Check sheet for the modelled part. Datum: model origin and axes. Units: mm. Face numbers are marked on the shaded views. A direction names the side the tool comes from. Round coordinates to 2 decimals unless told otherwise and drop trailing zeros. Write each loop counter-clockwise with the first axis right and the second up, starting at its lowest first coordinate (ties: lowest second). Pieces come first, ordered by that corner, then holes. Notation, with made-up numbers: (-36.75, 82) -> (2.25, 82) arc R24 cw to (2.25, 112) -> close; hole circle Ø3 at (51, -33.75). An arc over 180 degrees is marked (long way). Answer as a JSON object with one key per item and string values. Group by question number.
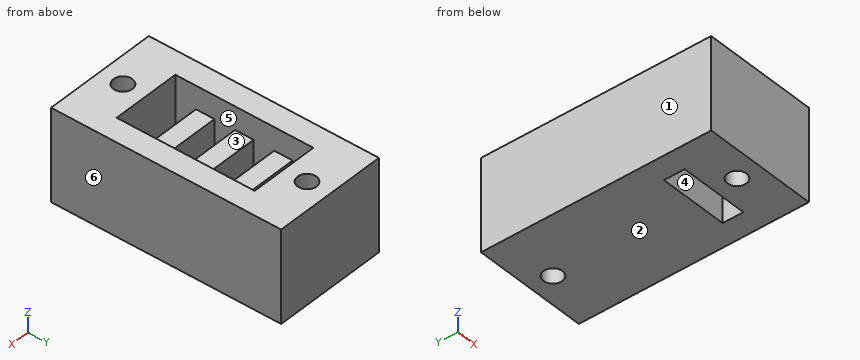
```python
from build123d import *

# Parameters (mm, degrees)
SKETCH1_W           = 12.7
SKETCH1_H           = 10.16
BOSS_EXTRUDE1_DEPTH = 25.4
SKETCH2_W           = 7.62
SKETCH2_H           = 15.24
CUT_EXTRUDE1_DEPTH  = 7.62
SKETCH3_W           = 5.08
SKETCH3_H           = 2.032
BOSS_EXTRUDE2_DEPTH = 7.62
SKETCH4_W           = 7.62
SKETCH4_H           = 2.286
CUT_EXTRUDE2_DEPTH  = 3.54
SKETCH5_R           = 1.0414
CUT_EXTRUDE4_DEPTH  = 11.16


with BuildPart() as part:
    # Sketch1 → Boss-Extrude1 (new body)
    with BuildSketch(Plane(origin=(0, 0, 0), x_dir=(1, 0, 0), z_dir=(0, 1, 0))):
        Rectangle(SKETCH1_W, SKETCH1_H)
    extrude(amount=BOSS_EXTRUDE1_DEPTH)

    # Sketch2 → Cut-Extrude1 (cut)
    with BuildSketch(Plane.XY.offset(5.08)):
        with Locations((0, 12.7)):
            Rectangle(SKETCH2_W, SKETCH2_H)
    extrude(amount=-CUT_EXTRUDE1_DEPTH, mode=Mode.SUBTRACT)

    # Sketch3 → Boss-Extrude2 (add)
    with BuildSketch(Plane.ZY.offset(-3.81)):
        with Locations((0, 12.7)):
            Rectangle(SKETCH3_W, SKETCH3_H)
        with Locations((0, 8.382)):
            Rectangle(SKETCH3_W, SKETCH3_H)
        with Locations((0, 17.018)):
            Rectangle(SKETCH3_W, SKETCH3_H)
    extrude(amount=BOSS_EXTRUDE2_DEPTH)

    # Sketch4 → Cut-Extrude2 (cut, through all)
    with BuildSketch(Plane.XY.offset(-2.54)):
        with Locations((0, 6.223)):
            Rectangle(SKETCH4_W, SKETCH4_H)
    extrude(amount=-CUT_EXTRUDE2_DEPTH, mode=Mode.SUBTRACT)

    # Sketch5 → Cut-Extrude4 (cut, through all)
    with BuildSketch(Plane.XY.offset(5.08)):
        with Locations((0, 2.54)):
            Circle(SKETCH5_R)
        with Locations((0, 22.86)):
            Circle(SKETCH5_R)
    extrude(amount=-CUT_EXTRUDE4_DEPTH, mode=Mode.SUBTRACT)


solid = part.part
```
(1) Section check A-A on x = 0. Record the cut outline in (y, z).
(2) Section check C-C on x = 3.5. Record the cut outline in (y, z), then the cut area to 3 significant figures.
(3) Access from +Z, -Z, +X, -X, +Y, -Y to the whole of each face (thin tool, end or side, straight path). Record for the marked faces 4, 5 and 6.
(4) Section check D-D on y = 2.54. Record the cut outline in (x, z).
(5) Release check for a two-part mould opening along X. For the marked faces 1, 2 and 3 record: pulls with the +X half, pulls with the -X half, needs draft (parallel to the pull), parting line crosses it, or undercut.
(6) Section check B-B on z = -1.25. Record the cut outline in (x, y), then the cut area to 3 significant figures.
(7) Scan lines: line 1 along Y through (x, z) = (0, 3.25); line 2 along Y through (x, z) = (-1.25, 3.5); line 3 along X through (y, z) = (15.5, -1). Record each from-to range of solid material in increasing order.
(8) Go/stop test with a flat-tipped pin: pin 1 Ø1.6 at (x, y) = (-1, 17.5) entering from +Z. Record where the tip stops, or that it passes through.
Data:
{
 "1": {"outline": "(0, -5.08) -> (1.5, -5.08) -> (1.5, 5.08) -> (0, 5.08) -> close; (3.58, -5.08) -> (5.08, -5.08) -> (5.08, 5.08) -> (3.58, 5.08) -> close; (7.37, -5.08) -> (21.82, -5.08) -> (21.82, 5.08) -> (20.32, 5.08) -> (20.32, -2.54) -> (18.03, -2.54) -> (18.03, 2.54) -> (16, 2.54) -> (16, -2.54) -> (13.72, -2.54) -> (13.72, 2.54) -> (11.68, 2.54) -> (11.68, -2.54) -> (9.4, -2.54) -> (9.4, 2.54) -> (7.37, 2.54) -> close; (23.9, -5.08) -> (25.4, -5.08) -> (25.4, 5.08) -> (23.9, 5.08) -> close"},
 "2": {"outline": "(0, -5.08) -> (5.08, -5.08) -> (5.08, 5.08) -> (0, 5.08) -> close; (7.37, -5.08) -> (25.4, -5.08) -> (25.4, 5.08) -> (20.32, 5.08) -> (20.32, -2.54) -> (18.03, -2.54) -> (18.03, 2.54) -> (16, 2.54) -> (16, -2.54) -> (13.72, -2.54) -> (13.72, 2.54) -> (11.68, 2.54) -> (11.68, -2.54) -> (9.4, -2.54) -> (9.4, 2.54) -> (7.37, 2.54) -> close", "area": "167 mm²"},
 "3": {"face 4": "+Z, -Z", "face 5": "+Z", "face 6": "+Z, -Z, +X, +Y, -Y"},
 "4": {"outline": "(-6.35, -5.08) -> (-1.04, -5.08) -> (-1.04, 5.08) -> (-6.35, 5.08) -> close; (1.04, -5.08) -> (6.35, -5.08) -> (6.35, 5.08) -> (1.04, 5.08) -> close"},
 "5": {"face 1": "pulls with the -X half", "face 2": "needs draft", "face 3": "undercut"},
 "6": {"outline": "(-6.35, 0) -> (6.35, 0) -> (6.35, 25.4) -> (-6.35, 25.4) -> close; hole (-3.81, 5.08) -> (3.81, 5.08) -> (3.81, 7.37) -> (-3.81, 7.37) -> close; hole (-3.81, 9.4) -> (3.81, 9.4) -> (3.81, 11.68) -> (-3.81, 11.68) -> close; hole (-3.81, 13.72) -> (3.81, 13.72) -> (3.81, 16) -> (-3.81, 16) -> close; hole (-3.81, 18.03) -> (3.81, 18.03) -> (3.81, 20.32) -> (-3.81, 20.32) -> close; hole circle Ø2.08 at (0, 2.54); hole circle Ø2.08 at (0, 22.86)", "area": "246 mm²"},
 "7": {"line 1": "y = 0 to 1.5, 3.58 to 5.08, 20.32 to 21.82, 23.9 to 25.4", "line 2": "y = 0 to 5.08, 20.32 to 25.4", "line 3": "x = -6.35 to -3.81, 3.81 to 6.35"},
 "8": {"pin 1": "stops at z = 2.54"}
}
